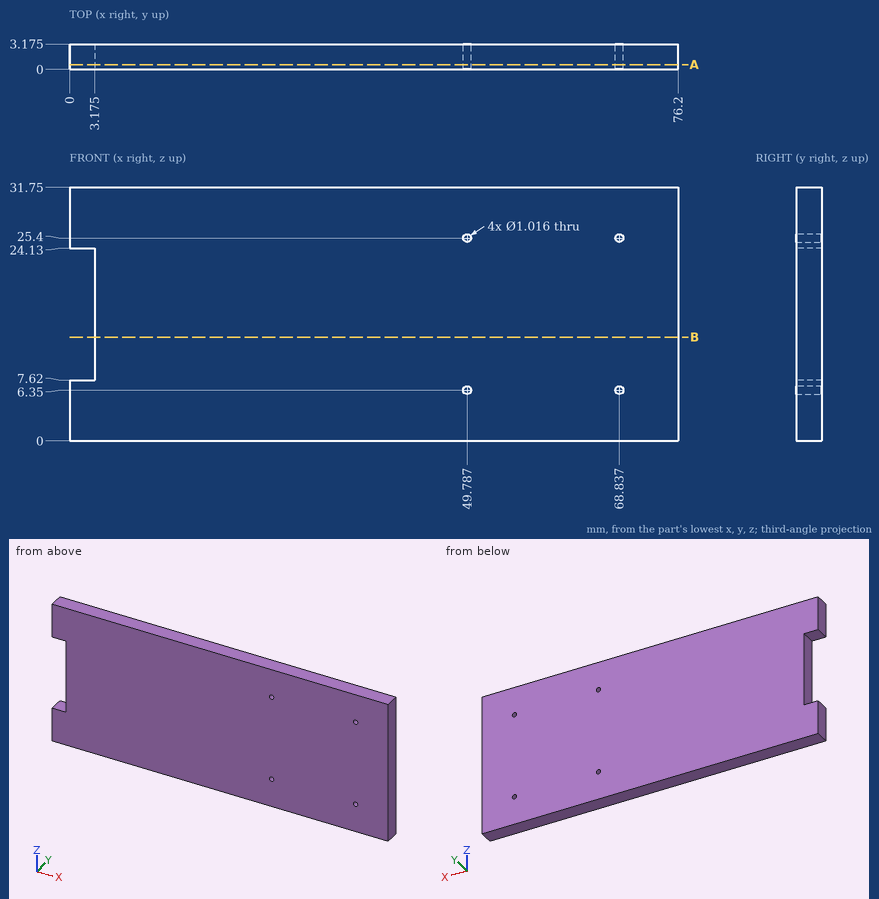
Source: three-view drawing plus pictorial views. Frame: mm from the lowest corner of the part. Round coordinates to 2 decimals unless told otherwise and drop trailing zeros. Order: outer loops, then holes, each group sorted by start corner. A loop starts at its lowest first (then second) coordinate and runs counter-clockwise, first axis right, second up. Notation, with made-up numbers: (-1.75, 22) - (29.25, 22) arc R17 ccw to (29.25, 52) - close; hole circle Ø7 at (18, 34). An arc over 180 degrees is marked (long way). Use a Markdown table: item, result.
1. Section A-A on y = 0.6. Return the cut outline in (x, z) (3 decimals), then the cut area to 3 significant figures.
Evaluation:
| item | result |
|---|---|
| outline | (0, 0) - (76.2, 0) - (76.2, 31.75) - (0, 31.75) - (0, 24.13) - (3.175, 24.13) - (3.175, 7.62) - (0, 7.62) - close; hole circle Ø1.016 at (49.787, 6.35); hole circle Ø1.016 at (49.787, 25.4); hole circle Ø1.016 at (68.837, 6.35); hole circle Ø1.016 at (68.837, 25.4) |
| area | 2,360 mm^2 |
2. Material intervals for probe 1 along X at (y, z) = (1.7, 6.35) (3 decimals); probe 2 along X at (y, z) = (0.6, 6); probe 3 along Z at (x, y) = (69, 2), sorted ascending.
Evaluation:
| item | result |
|---|---|
| probe 1 | 0 to 49.279, 50.295 to 68.329, 69.345 to 76.2 |
| probe 2 | 0 to 49.42, 50.16 to 68.47, 69.21 to 76.2 |
| probe 3 | 0 to 5.87, 6.83 to 24.92, 25.88 to 31.75 |
3. Section B-B on z = 13. Return the cut outline in (x, y) (3 decimals).
Evaluation:
| item | result |
|---|---|
| outline | (3.175, 0) - (76.2, 0) - (76.2, 3.175) - (3.175, 3.175) - close |
4. First-contact query: pin 1 (1.6 mm diameter, centred on x = 2, y = 1.5, fed in from -Z); pin 2 (1.6 mm diameter, centred on y = 1.5, z = 14.5, fed in from -X) (3 decimals). Flat tips, straight axial feed; report the tip coordinate or a pass-through.
Evaluation:
| item | result |
|---|---|
| pin 1 | z = 0 |
| pin 2 | x = 3.175 |
